from build123d import *

# Parameters (mm, degrees)
BOSS_EXTRUDE1_DEPTH             = 3.0734
L_BRACKET_MOUNT_HOLES_8_D       = 4.4958
SKETCH6_R                       = 6.35
ATLAS_SENSORS_DEPTH             = 4.0734
ATLAS_SENSOR_PATTERN_COUNT      = 3
ATLAS_SENSOR_PATTERN_PITCH      = 25.4
ATLAS_SENSOR_PATTERN_COUNT_DIR2 = 2
ATLAS_SENSOR_PATTERN_PITCH_DIR2 = 25.4
NUTRIENT_START                  = -4.0734
SKETCH7_R                       = 3.0226
NUTRIENT_HOSES_DEPTH            = 5.0734
LPATTERN2_COUNT                 = 2
LPATTERN2_PITCH                 = 12.7
LPATTERN2_COUNT_DIR2            = 5
LPATTERN2_PITCH_DIR2            = 12.7
WATER_LEVEL_SENSOR_D            = 4.4958
TEMP_SENSOR_MOUNTING_DEPTH      = 4.0734
SKETCH12_W                      = 38.1
SKETCH12_H                      = 50.8
ACCESSORY_HOLE_DEPTH            = 4.0734
FILLET1_R                       = 2.54
F_8_CLEARANCE_HOLE3_D           = 4.4958
LPATTERN3_COUNT                 = 2
LPATTERN3_PITCH                 = 62.23
FILLET1_OF_LPATTERN3_R          = 2.54
PUMP_WIRE_ZIP_TIE_DEPTH         = 4.0734
WIRE_ZIP_TIE_DEPTH              = 4.0734
LPATTERN4_COUNT                 = 2
LPATTERN4_PITCH                 = 55.88
F_1_4_CLEARANCE_HOLE1_D         = 6.5278


with BuildPart() as part:
    # Sketch1 → Boss-Extrude1 (new body)
    with BuildSketch(Plane(origin=(0, 0, 0), x_dir=(1, 0, 0), z_dir=(0, 1, 0))):
        with BuildLine():
            Line((0, 0), (381, 0))
            Line((381, 0), (381, 55.5625))
            ThreePointArc((381, 55.5625), (367.050960454, 89.238460454), (333.375, 103.1875))
            Line((333.375, 103.1875), (47.625, 103.1875))
            ThreePointArc((47.625, 103.1875), (13.949039546, 89.238460454), (0, 55.5625))
            Line((0, 55.5625), (0, 0))
        make_face()
    extrude(amount=BOSS_EXTRUDE1_DEPTH)

    # L Bracket Mount Holes (#8) (through all)
    with Locations(Plane(origin=(0, 3.0734, 0), x_dir=(1, 0, 0), z_dir=(0, 1, 0))):
        with Locations((38.1, 13.8557), (342.9, 13.8557), (53.975, 67.1068), (327.025, 67.1068), (190.5, 13.8557)):
            Hole(L_BRACKET_MOUNT_HOLES_8_D / 2)

    # Sketch6 → Atlas Sensors (cut, through all)
    with BuildSketch(Plane(origin=(0, 3.0734, 0), x_dir=(1, 0, 0), z_dir=(0, 1, 0))):
        with Locations((304.8, 65.0875)):
            Circle(SKETCH6_R)
    atlas_sensors = extrude(amount=-ATLAS_SENSORS_DEPTH, mode=Mode.SUBTRACT)

    # Atlas Sensor Pattern: Atlas Sensors 3 × 2
    with Locations(*[(-j * ATLAS_SENSOR_PATTERN_PITCH_DIR2, 0, i * ATLAS_SENSOR_PATTERN_PITCH) for i in range(ATLAS_SENSOR_PATTERN_COUNT) for j in range(ATLAS_SENSOR_PATTERN_COUNT_DIR2) if (i, j) != (0, 0)]):
        add(atlas_sensors, mode=Mode.SUBTRACT)

    # Sketch7 → Nutrient Hoses (cut)
    with BuildSketch(Plane(origin=(0, 3.0734, 0), x_dir=(1, 0, 0), z_dir=(0, 1, 0)).offset(NUTRIENT_START)):
        with Locations((260.35, 65.0875)):
            Circle(SKETCH7_R)
    nutrient_hoses = extrude(amount=NUTRIENT_HOSES_DEPTH, mode=Mode.SUBTRACT)

    # LPattern2: Nutrient Hoses 2 × 5
    with Locations(*[(-i * LPATTERN2_PITCH, 0, j * LPATTERN2_PITCH_DIR2) for i in range(LPATTERN2_COUNT) for j in range(LPATTERN2_COUNT_DIR2) if (i, j) != (0, 0)]):
        add(nutrient_hoses, mode=Mode.SUBTRACT)

    # Water Level Sensor (through all)
    with Locations(Plane(origin=(0, 3.0734, 0), x_dir=(1, 0, 0), z_dir=(0, 1, 0))):
        with Locations((234.95, 60.9473), (234.95, 39.6875), (234.95, 73.6473)):
            Hole(WATER_LEVEL_SENSOR_D / 2)

    # Sketch10 → temp sensor mounting (cut, through all)
    with BuildSketch(Plane(origin=(0, 3.0734, 0), x_dir=(1, 0, 0), z_dir=(0, 1, 0))):
        with BuildLine():
            Line((321.46875, 9.779), (321.46875, 15.621))
            ThreePointArc((321.46875, 15.621), (321.543144878, 15.800605122), (321.72275, 15.875))
            Line((321.72275, 15.875), (323.596, 15.875))
            ThreePointArc((323.596, 15.875), (323.775605122, 15.800605122), (323.85, 15.621))
            Line((323.85, 15.621), (323.85, 9.779))
            ThreePointArc((323.85, 9.779), (323.775605122, 9.599394878), (323.596, 9.525))
            Line((323.596, 9.525), (321.72275, 9.525))
            ThreePointArc((321.72275, 9.525), (321.543144878, 9.599394878), (321.46875, 9.779))
        make_face()
        with BuildLine():
            Line((326.644, 9.525), (328.51725, 9.525))
            ThreePointArc((328.51725, 9.525), (328.696855122, 9.599394878), (328.77125, 9.779))
            Line((328.77125, 9.779), (328.77125, 15.621))
            ThreePointArc((328.77125, 15.621), (328.696855122, 15.800605122), (328.51725, 15.875))
            Line((328.51725, 15.875), (326.644, 15.875))
            ThreePointArc((326.644, 15.875), (326.464394878, 15.800605122), (326.39, 15.621))
            Line((326.39, 15.621), (326.39, 9.779))
            ThreePointArc((326.39, 9.779), (326.464394878, 9.599394878), (326.644, 9.525))
        make_face()
        with BuildLine():
            Line((318.643, 30.48), (318.643, 33.02))
            ThreePointArc((318.643, 33.02), (325.12, 39.497), (331.597, 33.02))
            Line((331.597, 33.02), (331.597, 30.48))
            ThreePointArc((331.597, 30.48), (325.12, 24.003), (318.643, 30.48))
        make_face()
    extrude(amount=-TEMP_SENSOR_MOUNTING_DEPTH, mode=Mode.SUBTRACT)

    # Sketch12 → Accessory Hole (cut, through all)
    with BuildSketch(Plane(origin=(0, 3.0734, 0), x_dir=(1, 0, 0), z_dir=(0, 1, 0))):
        with Locations((152.4, 38.1)):
            Rectangle(SKETCH12_W, SKETCH12_H)
    accessory_hole = extrude(amount=-ACCESSORY_HOLE_DEPTH, mode=Mode.SUBTRACT)

    # Fillet1
    fillet1_edges = [part.edges().sort_by_distance(p)[0] for p in [
        (133.35, 1.5367, -12.7),
        (133.35, 1.5367, -63.5),
        (171.45, 1.5367, -63.5),
        (171.45, 1.5367, -12.7),
    ]]
    fillet(fillet1_edges, radius=FILLET1_R)

    # #8 Clearance Hole3 (through all)
    with Locations(Plane(origin=(0, 3.0734, 0), x_dir=(1, 0, 0), z_dir=(0, 1, 0))):
        with Locations((128.524, 68.326), (176.276, 68.326), (176.276, 7.874), (128.524, 7.874)):
            f_8_clearance_hole3 = Hole(F_8_CLEARANCE_HOLE3_D / 2)

    # LPattern3: Accessory Hole, #8 Clearance Hole3 ×2
    with Locations(*[(-i * LPATTERN3_PITCH, 0, 0) for i in range(1, LPATTERN3_COUNT)]):
        add(accessory_hole, mode=Mode.SUBTRACT)
        add(f_8_clearance_hole3, mode=Mode.SUBTRACT)

    # Fillet1 of LPattern3
    fillet1_of_lpattern3_edges = [part.edges().sort_by_distance(p)[0] for p in [
        (71.12, 1.5367, -12.7),
        (71.12, 1.5367, -63.5),
        (109.22, 1.5367, -63.5),
        (109.22, 1.5367, -12.7),
    ]]
    fillet(fillet1_of_lpattern3_edges, radius=FILLET1_OF_LPATTERN3_R)

    # Sketch16 → Pump Wire zip tie (cut, through all)
    with BuildSketch(Plane(origin=(0, 3.0734, 0), x_dir=(1, 0, 0), z_dir=(0, 1, 0))):
        with BuildLine():
            Line((212.50275, 15.875), (214.376, 15.875))
            ThreePointArc((214.376, 15.875), (214.555605122, 15.800605122), (214.63, 15.621))
            Line((214.63, 15.621), (214.63, 9.779))
            ThreePointArc((214.63, 9.779), (214.555605122, 9.599394878), (214.376, 9.525))
            Line((214.376, 9.525), (212.50275, 9.525))
            ThreePointArc((212.50275, 9.525), (212.323144878, 9.599394878), (212.24875, 9.779))
            Line((212.24875, 9.779), (212.24875, 15.621))
            ThreePointArc((212.24875, 15.621), (212.323144878, 15.800605122), (212.50275, 15.875))
        make_face()
        with BuildLine():
            Line((219.29725, 9.525), (217.424, 9.525))
            ThreePointArc((217.424, 9.525), (217.244394878, 9.599394878), (217.17, 9.779))
            Line((217.17, 9.779), (217.17, 15.621))
            ThreePointArc((217.17, 15.621), (217.244394878, 15.800605122), (217.424, 15.875))
            Line((217.424, 15.875), (219.29725, 15.875))
            ThreePointArc((219.29725, 15.875), (219.476855122, 15.800605122), (219.55125, 15.621))
            Line((219.55125, 15.621), (219.55125, 9.779))
            ThreePointArc((219.55125, 9.779), (219.476855122, 9.599394878), (219.29725, 9.525))
        make_face()
    extrude(amount=-PUMP_WIRE_ZIP_TIE_DEPTH, mode=Mode.SUBTRACT)

    # Sketch18 → Wire Zip Tie (cut, through all)
    with BuildSketch(Plane(origin=(0, 3.0734, 0), x_dir=(1, 0, 0), z_dir=(0, 1, 0))):
        with BuildLine():
            Line((273.304, 89.05875), (279.146, 89.05875))
            ThreePointArc((279.146, 89.05875), (279.325605122, 88.984355122), (279.4, 88.80475))
            Line((279.4, 88.80475), (279.4, 86.9315))
            ThreePointArc((279.4, 86.9315), (279.325605122, 86.751894878), (279.146, 86.6775))
            Line((279.146, 86.6775), (273.304, 86.6775))
            ThreePointArc((273.304, 86.6775), (273.124394878, 86.751894878), (273.05, 86.9315))
            Line((273.05, 86.9315), (273.05, 88.80475))
            ThreePointArc((273.05, 88.80475), (273.124394878, 88.984355122), (273.304, 89.05875))
        make_face()
        with BuildLine():
            Line((279.4, 82.01025), (279.4, 83.8835))
            ThreePointArc((279.4, 83.8835), (279.325605122, 84.063105122), (279.146, 84.1375))
            Line((279.146, 84.1375), (273.304, 84.1375))
            ThreePointArc((273.304, 84.1375), (273.124394878, 84.063105122), (273.05, 83.8835))
            Line((273.05, 83.8835), (273.05, 82.01025))
            ThreePointArc((273.05, 82.01025), (273.124394878, 81.830644878), (273.304, 81.75625))
            Line((273.304, 81.75625), (279.146, 81.75625))
            ThreePointArc((279.146, 81.75625), (279.325605122, 81.830644878), (279.4, 82.01025))
        make_face()
    wire_zip_tie = extrude(amount=-WIRE_ZIP_TIE_DEPTH, mode=Mode.SUBTRACT)

    # LPattern4: Wire Zip Tie ×2
    with Locations(*[(-i * LPATTERN4_PITCH, 0, 0) for i in range(1, LPATTERN4_COUNT)]):
        add(wire_zip_tie, mode=Mode.SUBTRACT)

    # 1/4 Clearance Hole1 (through all)
    with Locations(Plane(origin=(0, 3.0734, 0), x_dir=(1, 0, 0), z_dir=(0, 1, 0))):
        with Locations((190.5, 32.9057)):
            Hole(F_1_4_CLEARANCE_HOLE1_D / 2)


solid = part.part
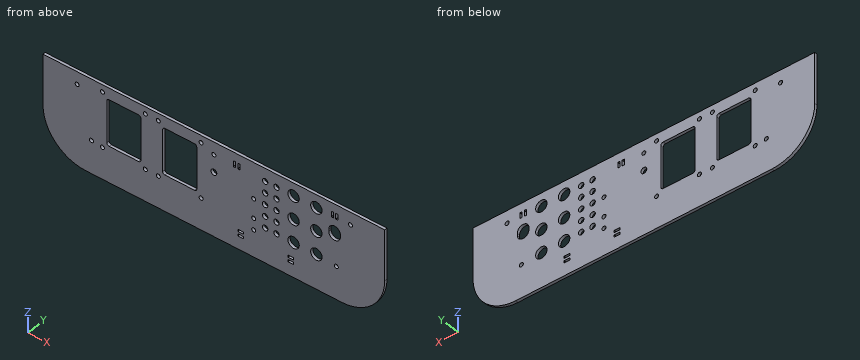
Read the model definition and answer for the solid it produces. Units are mm, in the model's axes. Round coordinates to 2 decimals unless told otherwise and drop trailing zeros. Order: outer loops, then holes, each group sorted by start corner. A loop starts at its lowest first (then second) coordinate and runs counter-clockwise, first axis right, second up.
1) Straight lines are drawn through the part: L1, parallel to Z at x = 247.65, y = 1.3; L2, parallel to X at y = 1.85, z = -46.5; L3, parallel to Z at x = 128, y = 1.3. For each, find the intervals that lie inside material, in ascending order.
2) The part is cut by section A-A on x = 164. Write down the section's boundary in (y, z).
3) Flat-ended cylindrical pins translate along their axes: pin 1 (3.5 mm diameter, centred on x = 247.65, z = -65.09, fed in from +Y); pin 2 (1.5 mm diameter, centred on y = 2, z = -88, fed in from -X); pin 3 (1.5 mm diameter, centred on y = 2, z = -87.5, fed in from +X). Find the tip coordinate at first contact, or state that the pin passes through.
4) The part is cut by section B-B on y = 2.5. Give the number of separate pieces and of enclosed holes in the cut face, plus the area to 3 significant figures.
Resolved:
1. L1: z = -103.19 to -68.11, -62.06 to -55.41, -49.36 to -42.71, -36.66 to -30.01, -23.96 to -17.31, -11.26 to 0
1. L2: x = 0 to 71.12, 109.22 to 133.35, 171.45 to 381
1. L3: z = -103.19 to -70.51, -66.14 to -10.06, -5.69 to 0
2. outline: (0, -103.19) - (3.07, -103.19) - (3.07, -63.5) - (0, -63.5) - close; (0, -12.7) - (3.07, -12.7) - (3.07, 0) - (0, 0) - close
3. pin 1: passes through
3. pin 2: stops at x = 12.07
3. pin 3: stops at x = 369.37
4. separate pieces: 1
4. enclosed holes: 44
4. area: 32,900 mm2
